Autodesk Inventor part; units mm, degrees
ref_plane "Start Plane" through (0, 0, 0) normal (0, 0, 1) x (1, 0, 0)
ref_plane "End Plane" through (0, 0, 20) normal (0, 0, 1) x (1, 0, 0)
ref_plane "YZ Plane" through (0, 0, 0) normal (1, 0, 0) x (0, 1, 0)
sketch "Sketch1" plane through (0, 0, 0) normal (0, 0, 1) x (1, 0, 0)
  line L0 (10, -4.5951) -> (10, -8.2)
  line L1 (-10, -8.2) -> (-10, -4.5951)
  line L2 (-10, 10) -> (10, -10) construction
  line L3 (10, 10) -> (-10, -10) construction
  circle A0 centre (0, 0) radius 2.1
  line L4 (-2.84, -3.9007) -> (2.84, -3.9007)
  line L5 (3.9007, -2.84) -> (3.9007, 2.84)
  line L6 (2.84, 3.9007) -> (-2.84, 3.9007)
  line L7 (-3.9007, 2.84) -> (-3.9007, -2.84)
  line L8 (-3.9007, -3.9007) -> (3.9007, 3.9007) construction
  line L9 (3.9007, -3.9007) -> (-3.9007, 3.9007) construction
  line L10 (-3.9007, -2.84) -> (-2.84, -3.9007) construction
  line L11 (-2.84, -3.9007) -> (-5.4993, -6.56)
  line L12 (-5.4993, -6.56) -> (-5.4993, -8.2)
  line L13 (-5.4993, -8.2) -> (-2.7951, -8.2)
  line L14 (-2.7951, -8.2) -> (-4.5951, -10)
  line L15 (0, 0) -> (0, -3.9007) construction
  line L16 (3.9007, -2.84) -> (2.84, -3.9007) construction
  line L17 (2.84, -3.9007) -> (5.4993, -6.56)
  line L18 (5.4993, -6.56) -> (5.4993, -8.2)
  line L19 (5.4993, -8.2) -> (2.7951, -8.2)
  line L20 (2.7951, -8.2) -> (4.5951, -10)
  line L21 (-2.84, -3.9007) -> (-3.9007, -2.84) construction
  line L22 (-3.9007, -2.84) -> (-6.56, -5.4993)
  line L23 (-6.56, -5.4993) -> (-8.2, -5.4993)
  line L24 (-8.2, -5.4993) -> (-8.2, -2.7951)
  line L25 (-8.2, -2.7951) -> (-10, -4.5951)
  line L26 (3.9007, -2.84) -> (6.56, -5.4993)
  line L27 (6.56, -5.4993) -> (8.2, -5.4993)
  line L28 (8.2, -5.4993) -> (8.2, -2.7951)
  line L29 (8.2, -2.7951) -> (10, -4.5951)
  arc A1 (-10, -8.2) -> (-8.2, -10) centre (-8.2, -8.2) ccw
  arc A2 (8.2, -10) -> (10, -8.2) centre (8.2, -8.2) ccw
  line L30 (-8.2, -6.56) -> (-7.7111, -6.56)
  line L31 (-6.6505, -8.2) -> (-8.2, -8.2)
  line L32 (-8.2, -8.2) -> (-8.2, -6.56)
  line L33 (-6.6505, -7.6207) -> (-7.7111, -6.56)
  line L34 (-6.6505, -7.6207) -> (-6.6505, -8.2)
  line L35 (8.2, -6.56) -> (7.7111, -6.56)
  line L36 (6.6505, -8.2) -> (8.2, -8.2)
  line L37 (8.2, -8.2) -> (8.2, -6.56)
  line L38 (6.6505, -7.6207) -> (7.7111, -6.56)
  line L39 (6.6505, -7.6207) -> (6.6505, -8.2)
  line L40 (8.2, -10) -> (4.5951, -10)
  line L41 (-4.5951, -10) -> (-8.2, -10)
  line L42 (-3.9007, 0) -> (3.9007, 0) construction
  line L43 (10, 4.5951) -> (10, 8.2)
  line L44 (-10, 8.2) -> (-10, 4.5951)
  line L45 (-2.84, 3.9007) -> (2.84, 3.9007)
  line L46 (-3.9007, 2.84) -> (-2.84, 3.9007) construction
  line L47 (-2.84, 3.9007) -> (-5.4993, 6.56)
  line L48 (-5.4993, 6.56) -> (-5.4993, 8.2)
  line L49 (-5.4993, 8.2) -> (-2.7951, 8.2)
  line L50 (-2.7951, 8.2) -> (-4.5951, 10)
  line L51 (2.84, 3.9007) -> (5.4993, 6.56)
  line L52 (5.4993, 6.56) -> (5.4993, 8.2)
  line L53 (5.4993, 8.2) -> (2.7951, 8.2)
  line L54 (2.7951, 8.2) -> (4.5951, 10)
  line L55 (3.9007, 2.84) -> (2.84, 3.9007) construction
  line L56 (-8.2, 2.7951) -> (-10, 4.5951)
  line L57 (-2.84, 3.9007) -> (-3.9007, 2.84) construction
  line L58 (-3.9007, 2.84) -> (-6.56, 5.4993)
  line L59 (-6.56, 5.4993) -> (-8.2, 5.4993)
  line L60 (-8.2, 5.4993) -> (-8.2, 2.7951)
  line L61 (3.9007, 2.84) -> (6.56, 5.4993)
  line L62 (6.56, 5.4993) -> (8.2, 5.4993)
  line L63 (8.2, 5.4993) -> (8.2, 2.7951)
  line L64 (8.2, 2.7951) -> (10, 4.5951)
  arc A3 (-8.2, 10) -> (-10, 8.2) centre (-8.2, 8.2) ccw
  arc A4 (10, 8.2) -> (8.2, 10) centre (8.2, 8.2) ccw
  line L65 (-8.2, 6.56) -> (-7.7111, 6.56)
  line L66 (-6.6505, 8.2) -> (-8.2, 8.2)
  line L67 (-8.2, 8.2) -> (-8.2, 6.56)
  line L68 (-6.6505, 7.6207) -> (-7.7111, 6.56)
  line L69 (-6.6505, 7.6207) -> (-6.6505, 8.2)
  line L70 (8.2, 6.56) -> (7.7111, 6.56)
  line L71 (6.6505, 7.6207) -> (7.7111, 6.56)
  line L72 (8.2, 8.2) -> (8.2, 6.56)
  line L73 (6.6505, 7.6207) -> (6.6505, 8.2)
  line L74 (6.6505, 8.2) -> (8.2, 8.2)
  line L75 (8.2, 10) -> (4.5951, 10)
  line L76 (-4.5951, 10) -> (-8.2, 10)
  line L77 (-8.2, 10) -> (-4.5951, 10)
  line L78 (4.5951, 10) -> (8.2, 10)
  point P0 (8.2, -8.2)
  point P1 (0, 3.9007)
  point P2 (8.2, 8.2)
  point P3 (0, 2.1)
  point P4 (1.4849, 1.4849)
  point P5 (0, 2.1)
  point P6 (0, 10)
  dimension "Width" = 20
  dimension "Height" = 20
  dimension "d2" = 4.2
  dimension "d3" = 1.5
  dimension "d4" = 1.64
  dimension "d6" = 5.68
  dimension "d7" = 1.8
  dimension "d9" = 1.5
ref_plane "Start Plane" through (0, 0, 0) normal (0, 0, 1) x (1, 0, 0)
ref_plane "End Plane" through (0, 0, 20) normal (0, 0, 1) x (1, 0, 0)
sketch "Sketch4" plane through (0, 0, 0) normal (0, 0, 1) x (1, 0, 0)
  line L0 (0, 0) -> (10, 0)
ref_plane "Work Plane4" through (0, 0, 0) normal (0, -1, 0) x (1, 0, 0)
sketch "Sketch5" plane through (0, 0, 0) normal (0, -1, 0) x (1, 0, 0)
  line L0 (-2, 0) -> (12, 0) construction
  line L1 (-2, 20) -> (12, 20) construction
  dimension "d17" = 20
extrude "Extrusion3" add sketch "Sketch1" along normal blind 150
equation "\"G_OFFSET_START\" = 0"
equation "\"G_OFFSET_END\" = 0"
equation "\"G_L\" = d17"
properties part number "V-slot 20 mm x 20 mm" material "Aluminum 6061"
The model under review builds one solid part; all positions refer to its coordinate system, in mm. A direction names the side the tool comes from. Round coordinates to 2 decimals unless told otherwise and drop trailing zeros. Write each loop counter-clockwise with the first axis right and the second up, starting at its lowest first coordinate (ties: lowest second). Pieces come first, ordered by that corner, then holes. Notation, with made-up numbers: M -16.75,5.5 L 9.25,5.5 A24 ccw 9.25,27.5 Z; hole C 68.25,4.5 d4. An arc over 180 degrees is marked long. Use a Markdown table: item, result. Add a question column.
Q1. We need section A-A, the plane y = 0. State the section outline as (x, z) points.
Q2. Machinability: for faces 4 (the face through (-6, 10, 74)), 5 (the face through (0, 3.901, 74)), 6 (the face through (-5.21, -4.15, 73.95)), which of the approach directions +Z, -Z, +X, -X, +Y, -Y give a long, thin tool a straight path to every point of the face, cutting with its end or side? Answer none if there is none.
Q3. Insertion check: pin 1 (1 mm diameter, centred on x = 1.5, z = 88.5, fed in from -Y); pin 2 (2 mm diameter, centred on y = -3.5, z = 92, fed in from +X); pin 3 (1.7 mm diameter, centred on y = 0, z = 94.5, fed in from +X). Each pin has a flat end and moves straight along its axis. Give the tip position at first contact, or say it passes through.
Q4. We need section C-C, the plane z = 21. Count the separate pieces of the cut face and the enclosed holes in it, plus the area to 3 significant figures.
Q5. To check wall thickness, follow line 1 (X direction, y = -3.5, z = 144.5); line 2 (Y direction, x = 0, z = 75.5); line 3 (Y direction, x = 4.25, z = 137.5). State the ranges of each line that lie inside material, in increasing order.
Q6. The part is to be moulded in two halves that separate along X. For faces 1 (the face through (-0.1, 2.4, 150)), 2 (the face through (3.901, 0, 74)), 3 (the face through (2.003, -0.631, 73.95)), say which applies: pulls with the +X half, pulls with the -X half, needs draft (parallel to the pull), parting line crosses it, or undercut.
Findings below:
| question | item | result |
|---|---|---|
| 1 | outline | M -3.9,0 L -2.1,0 L -2.1,150 L -3.9,150 Z; M 2.1,0 L 3.9,0 L 3.9,150 L 2.1,150 Z |
| 2 | face 4 | +Z, -Z, +X, -X, +Y |
| 2 | face 5 | +Z, -Z, +Y |
| 2 | face 6 | +Z, -Z |
| 3 | pin 1 | stops at y = -3.9 |
| 3 | pin 2 | stops at x = 9.9 |
| 3 | pin 3 | stops at x = 3.9 |
| 4 | separate pieces | 1 |
| 4 | enclosed holes | 5 |
| 4 | area | 161 mm² |
| 5 | line 1 | x = -8.9 to -8.2, -4.56 to 4.56, 8.2 to 8.9 |
| 5 | line 2 | y = -3.9 to -2.1, 2.1 to 3.9 |
| 5 | line 3 | y = -9.65 to -8.2, -5.31 to -3.19, 3.19 to 5.31, 8.2 to 9.65 |
| 6 | face 1 | needs draft |
| 6 | face 2 | pulls with the +X half |
| 6 | face 3 | undercut |
